Check sheet for the drawn part. Datum: minimum x, y, z corner. Units: mm. A direction names the side the tool comes from. Coordinates: 2 decimals unless noted, no trailing zeros. Write each loop counter-clockwise with the first axis right and the second up, starting at its lowest first coordinate (ties: lowest second). Pieces come first, ordered by that corner, then holes. Notation, with made-up numbers: M 18,46.5 L 29,46.5 A19 ccw 29,82.5 Z; hole C -20.75,29 d10. An arc over 180 degrees is marked long. Answer as CSV lines item,"result". Start each with the question number.
Q1. Access from +Z, -Z, +X, -X, +Y, -Y to the whole of each face (thin tool, end or side, straight path). Record for the marked faces 1, 2 and 3.
Q2. Sectioned sample at D-D, the plane x = 60. Record the cut outline in (y, z), then the cut area to 3 significant figures.
Q3. Sectioned sample at A-A, the plane x = 30. Record the cut outline in (y, z) (1 decimal).
Q4. Depth check by flat-ended pin: pin 1 Ø4 at (x, y) = (36.5, 44) entering from -Z; pin 2 Ø6.5 at (x, z) = (66.5, 3) entering from +Y (1 decimal); pin 3 Ø6 at (x, z) = (61.5, 9) entering from +Y (1 decimal). Enter the tip coordinate at first touch or a pass-through.
Q5. Thickness scan on line 1 along Y through (x, z) = (40.5, 8.75) (1 decimal); line 2 along X through (y, z) = (5.5, 3.25); line 3 along Z through (x, y) = (21.5, 44.5). Record the ranges inside material, lowest first. Write a range as from..to.
Q6. Sectioned sample at C-C, the plane y = 13. Record the cut outline in (x, z), then the cut area to 3 significant figures.
Q7. Sectioned sample at B-B, the plane z = 3.75. Count the separate pieces of the cut face and the enclosed holes in it, then the cut area to 3 significant figures.
Q8. Mould release check, pull along Y, two halves, no side actions. Record for the marked faces 4, 5, 6 and 7: pulls with the +Y half, pulls with the -Y half, needs draft (parallel to the pull), parting line crosses it, or undercut.
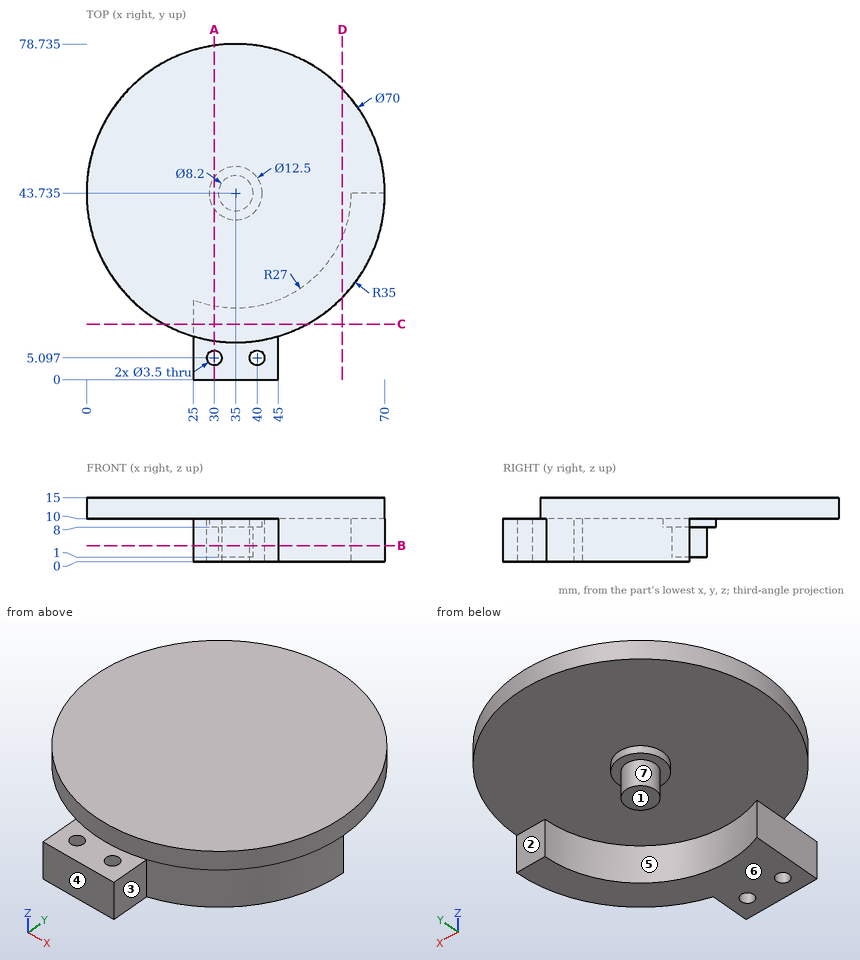
Output:
1,face 1,"-Z, -X, +Y"
1,face 2,"-Z, +X, +Y"
1,face 3,"+Z, -Z, +X, -Y"
2,outline,"M 19.24,0 L 33.54,0 L 33.54,10 L 68.23,10 L 68.23,15 L 19.24,15 Z"
2,area,"388 mm^2"
3,outline,"M 0,0 L 3.3,0 L 3.3,10 L 0,10 Z; M 6.8,0 L 17.2,0 L 17.2,10 L 40,10 L 40,8 L 47.5,8 L 47.5,10 L 78.4,10 L 78.4,15 L 9.1,15 L 9.1,10 L 6.8,10 Z"
4,pin 1,"stops at z = 1"
4,pin 2,"stops at y = 43.7"
4,pin 3,"stops at y = 69.5"
5,line 1,"y = 0..3.4, 6.8..17.3, 40.8..46.7"
5,line 2,"x = 25..28.3, 31.7..38.3, 41.7..45"
5,line 3,"z = 10..15"
6,outline,"M 18.26,10 L 25,10 L 25,0 L 51.74,0 L 51.74,15 L 18.26,15 Z"
6,area,"435 mm^2"
7,separate pieces,"2"
7,enclosed holes,"2"
7,area,"689 mm^2"
8,face 4,"pulls with the -Y half"
8,face 5,"undercut"
8,face 6,"needs draft"
8,face 7,"undercut"
